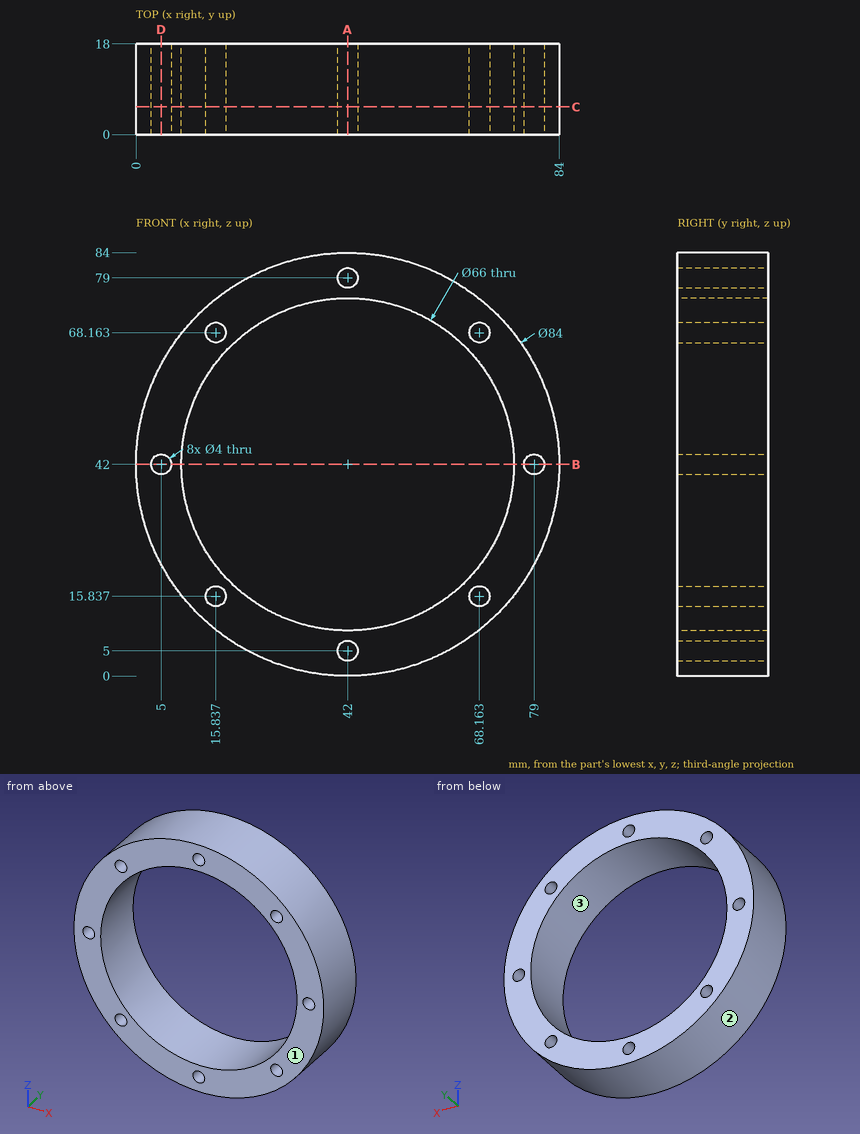
Study the drawing (mm; zero at the part's minimum x, y, z) and answer. Coordinates: 2 decimals unless noted, no trailing zeros. Write each loop counter-clockwise with the first axis right and the second up, starting at its lowest first coordinate (ties: lowest second). Pieces come first, ordered by that corner, then holes.
Q1. Determine the mould class of the marked faces 1, 2 and 3 for opening direction Z: released by +Z, released by -Z, zero draft, split by the parting line, or undercut.
Q2. Find the intervals of material crossed by line 1 (Z direction, x = 42, y = 13); line 2 (X direction, y = 2.25, z = 43); line 3 (X direction, y = 3, z = 15), in increasing order.
Q3. A cutting plane is placed at C-C, the plane y = 5.5. State how many separate pieces and enclosed holes the cut face has, then the cut area to 3 significant figures.
Q4. A cutting plane is placed at A-A, the plane x = 42. Give the vertices of the cut face in (y, z).
Q5. Each of these flat-tipped pins is pushed along its axis until it touches: pin 1 Ø2 at (y, z) = (9, 50.5) entering from -X; pin 2 Ø1 at (y, z) = (5.5, 74) entering from -X; pin 3 Ø6 at (y, z) = (15.5, 21) entering from +X; pin 4 Ø3.5 at (x, z) = (68.163, 15.837) entering from -Y. Where does it stop, or does it pass through?
Q6. A cutting plane is placed at B-B, the plane z = 42. Give the vertices of the cut face in (x, y).
Q7. A cutting plane is placed at D-D, the plane x = 5. Give the vertices of the cut face in (y, z), then the cut area to 3 significant figures.
Findings below:
1. face 1: zero draft
1. face 2: split by the parting line
1. face 3: undercut
2. line 1: z = 0 to 3, 7 to 9, 75 to 77, 81 to 84
2. line 2: x = 0.01 to 3.27, 6.73 to 9.02, 74.98 to 77.27, 80.73 to 83.99
2. line 3: x = 9.83 to 14.02, 17.65 to 23.03, 60.97 to 66.35, 69.98 to 74.17
3. separate pieces: 1
3. enclosed holes: 9
3. area: 2,020 mm2
4. outline: (0, 0) - (18, 0) - (18, 3) - (0, 3) - close; (0, 7) - (18, 7) - (18, 9) - (0, 9) - close; (0, 75) - (18, 75) - (18, 77) - (0, 77) - close; (0, 81) - (18, 81) - (18, 84) - (0, 84) - close
5. pin 1: stops at x = 0.68
5. pin 2: stops at x = 14.22
5. pin 3: stops at x = 79.95
5. pin 4: passes through
6. outline: (0, 0) - (3, 0) - (3, 18) - (0, 18) - close; (7, 0) - (9, 0) - (9, 18) - (7, 18) - close; (75, 0) - (77, 0) - (77, 18) - (75, 18) - close; (81, 0) - (84, 0) - (84, 18) - (81, 18) - close
7. outline: (0, 22.13) - (18, 22.13) - (18, 40) - (0, 40) - close; (0, 44) - (18, 44) - (18, 61.87) - (0, 61.87) - close
7. area: 643 mm2
